Work out the finished part from the listing and answer in its coordinate system (mm). Round coordinates to 2 decimals unless told otherwise and drop trailing zeros. Order: outer loops, then holes, each group sorted by start corner. A loop starts at its lowest first (then second) coordinate and runs counter-clockwise, first axis right, second up.
Autodesk Inventor part; units mm, degrees
ref_plane "YZ Plane" through (0, 0, 0) normal (1, 0, 0) x (0, 1, 0)
ref_plane "XZ Plane" through (0, 0, 0) normal (0, 1, 0) x (-1, 0, 0)
ref_plane "XY Plane" through (0, 0, 0) normal (0, 0, 1) x (1, 0, 0)
sketch "Sketch1" plane through (0, 0, 0) normal (0, 1, 0) x (-1, 0, 0)
  line L0 (0, 0) -> (-5.6352, 0)
  line L1 (-5.6352, 0) -> (0, 0)
  line L2 (0, 0) -> (0, 8.7024)
  line L3 (6.5, 14) -> (-6.5, 14)
  line L4 (-6.5, 14) -> (-6.5, 0)
  line L5 (-6.5, 0) -> (6.5, 0)
  line L6 (6.5, 0) -> (6.5, 14)
  circle A0 centre (0, -5) radius 1.5
  circle A1 centre (0, 19) radius 1.5
  line L7 (0, 19) -> (0, -5)
  line L8 (0, 19) -> (0, -5) construction
  line L9 (-10, 19) -> (-10, -5)
  line L10 (10, -5) -> (10, 19)
  arc A2 (10, 19) -> (-10, 19) centre (0, 19) ccw
  arc A3 (-10, -5) -> (10, -5) centre (0, -5) ccw
  point P0 (0, -8.7024)
  point P1 (0, 7)
  dimension "d25" = 13
  dimension "d26" = 14
  dimension "d30" = 5
  dimension "d31" = 5
  dimension "d32" = 3
  dimension "d33" = 20
extrude "Extrusion1" add sketch "Sketch1" along normal blind 6 contours L0 L5 L4 L3 L7 L2 | L2 L7 L3 L6 L5 | A2 L10 A3 L9
properties part number "case_usb_cap" material "Acrylic, Clear"
Item 1: For a pull along X with two mould halves and no side action, classify faces 1 (the face through (1.5, 2.96, -5.07)), 2 (the face through (0, 3, 29)), 3 (the face through (0, 0, 7)) as released by +X, released by -X, zero draft, split by the parting line, or undercut.
Item 2: Find section B-B (y = 1.7). Write down the section's boundary in (x, z), plus the area to 3 significant figures.
Item 3: Given pin 1 (2 mm diameter, centred on x = -2.5, y = 2.5, fed in from -Z); pin 2 (2.5 mm diameter, centred on x = 0, z = -5, fed in from +Y), each flat-ended and moving along its own axis, determine where each tip first touches the part or whether it passes through.
Item 4: Find the intervals of material crossed by line 1 along Z through (x, y) = (0, 1.85); line 2 along X through (y, z) = (1.5, -5); line 3 along X through (y, z) = (2.9, 18), in increasing order.
Item 5: Find section D-D (x = 8.25). Write down the section's boundary in (y, z).
Item 6: Find section C-C (x = -7.5). Write down the section's boundary in (y, z), plus the area to 3 significant figures.
Item 7: Find section A-A (x = 0). Write down the section's boundary in (y, z).
Model answer:
1. face 1: undercut
1. face 2: split by the parting line
1. face 3: zero draft
2. outline: (-10, -5) arc R10 ccw to (10, -5) - (10, 19) arc R10 ccw to (-10, 19) - close; hole circle Ø3 at (0, -5); hole circle Ø3 at (0, 19)
2. area: 780 mm2
3. pin 1: stops at z = -14.89
3. pin 2: passes through
4. line 1: z = -15 to -6.5, -3.5 to 17.5, 20.5 to 29
4. line 2: x = -10 to -1.5, 1.5 to 10
4. line 3: x = -10 to -1.12, 1.12 to 10
5. outline: (0, -10.65) - (6, -10.65) - (6, 24.65) - (0, 24.65) - close
6. outline: (0, -11.61) - (6, -11.61) - (6, 25.61) - (0, 25.61) - close
6. area: 223 mm2
7. outline: (0, -15) - (6, -15) - (6, -6.5) - (0, -6.5) - close; (0, -3.5) - (6, -3.5) - (6, 17.5) - (0, 17.5) - close; (0, 20.5) - (6, 20.5) - (6, 29) - (0, 29) - close
